```python
from build123d import *

# Parameters (mm, degrees)
BOSS_EXTRUDE1_DEPTH              = 5
SKETCH3_W                        = 11
SKETCH3_H                        = 5
BOSS_EXTRUDE2_DEPTH              = 5
SKETCH4_W                        = 5
SKETCH4_H                        = 5
BOSS_EXTRUDE3_DEPTH              = 21
SKETCH5_W                        = 10
SKETCH5_H                        = 5
BOSS_EXTRUDE4_DEPTH              = 20
SKETCH6_W                        = 11
SKETCH6_H                        = 5
BOSS_EXTRUDE5_DEPTH              = 5
SKETCH7_W                        = 5
SKETCH7_H                        = 5
BOSS_EXTRUDE6_DEPTH              = 21
SKETCH8_W                        = 10
SKETCH8_H                        = 5
BOSS_EXTRUDE7_DEPTH              = 20
SKETCH11_W                       = 10
SKETCH11_H                       = 5
BOSS_EXTRUDE8_DEPTH              = 3.5
SKETCH12_W                       = 10
SKETCH12_H                       = 5
BOSS_EXTRUDE9_DEPTH              = 3.5
CUT_EXTRUDE6_DEPTH               = 14.5
CUT_EXTRUDE8_DEPTH               = 41.078048855
CUT_EXTRUDE8_DEPTH_BACK          = 14.5
SKETCH17_W                       = 1.38
SKETCH17_H                       = 3.56
CUT_EXTRUDE9_DEPTH               = 14.5
CUT_EXTRUDE10_DEPTH              = 14.5
SKETCH_1_W                       = 8
SKETCH_1_H                       = 25
EXTRUDE_1_DEPTH                  = 5
SKETCH_2_W                       = 8
SKETCH_2_H                       = 25
EXTRUDE_2_DEPTH                  = 5
SKIZZE1_R                        = 1.5
SCHNITT_LINEAR_AUSTRAGEN1_DEPTH  = 10
AUFSATZ_LINEAR_AUSTRAGEN1_DEPTH  = 4
SKIZZE3_W                        = 10
SKIZZE3_H                        = 5
SCHNITT_LINEAR_AUSTRAGEN2_DEPTH  = 3.5
SCHNITT_LINEAR_AUSTRAGEN3_DEPTH  = 4
AUFSATZ_LINEAR_AUSTRAGEN3_DEPTH  = 11
SKIZZE7_R                        = 1.5
SCHNITT_LINEAR_AUSTRAGEN6_DEPTH  = 10
SKIZZE8_W                        = 10
SKIZZE8_H                        = 5
SCHNITT_LINEAR_AUSTRAGEN8_DEPTH  = 4
AUFSATZ_LINEAR_AUSTRAGEN4_DEPTH  = 4
SCHNITT_LINEAR_AUSTRAGEN9_DEPTH  = 4
AUFSATZ_LINEAR_AUSTRAGEN6_DEPTH  = 11
SKIZZE12_R                       = 1.5
SCHNITT_LINEAR_AUSTRAGEN10_DEPTH = 11


with BuildPart() as part:
    # Sketch1 → Boss-Extrude1 (new body)
    with BuildSketch(Plane(origin=(0, 0, 0), x_dir=(1, 0, 0), z_dir=(0, 1, 0))):
        Polygon((5.5, 3), (5.5, 0), (5.5, -3), (5.5, -8.5), (0, -8.5), (-5.5, -8.5), (-5.5, -3), (-5.5, 8.5), (0, 8.5), (5.5, 8.5), align=None)
    extrude(amount=BOSS_EXTRUDE1_DEPTH)

    # Sketch3 → Boss-Extrude2 (add)
    with BuildSketch(Plane.XY.offset(8.5)):
        with Locations((0, 2.5)):
            Rectangle(SKETCH3_W, SKETCH3_H)
    extrude(amount=BOSS_EXTRUDE2_DEPTH)

    # Sketch4 → Boss-Extrude3 (add)
    with BuildSketch(Plane(origin=(5.5, 0, 0), x_dir=(0, 0, -1), z_dir=(1, 0, 0))):
        with Locations((-11, 2.5)):
            Rectangle(SKETCH4_W, SKETCH4_H)
    extrude(amount=BOSS_EXTRUDE3_DEPTH)

    # Sketch5 → Boss-Extrude4 (add)
    with BuildSketch(Plane.XZ):
        with Locations((21.5, 11)):
            Rectangle(SKETCH5_W, SKETCH5_H)
    extrude(amount=BOSS_EXTRUDE4_DEPTH)

    # Sketch6 → Boss-Extrude5 (add)
    with BuildSketch(Plane(origin=(0, 0, -8.5), x_dir=(-1, 0, 0), z_dir=(0, 0, -1))):
        with Locations((0, 2.5)):
            Rectangle(SKETCH6_W, SKETCH6_H)
    extrude(amount=BOSS_EXTRUDE5_DEPTH)

    # Sketch7 → Boss-Extrude6 (add)
    with BuildSketch(Plane(origin=(5.5, 0, 0), x_dir=(0, 0, -1), z_dir=(1, 0, 0))):
        with Locations((11, 2.5)):
            Rectangle(SKETCH7_W, SKETCH7_H)
    extrude(amount=BOSS_EXTRUDE6_DEPTH)

    # Sketch8 → Boss-Extrude7 (add)
    with BuildSketch(Plane(origin=(0, 0, 0), x_dir=(-1, 0, 0), z_dir=(0, -1, 0))):
        with Locations((-21.5, 11)):
            Rectangle(SKETCH8_W, SKETCH8_H)
    extrude(amount=BOSS_EXTRUDE7_DEPTH)

    # Sketch11 → Boss-Extrude8 (add)
    with BuildSketch(Plane(origin=(0, 0, 8.5), x_dir=(-1, 0, 0), z_dir=(0, 0, -1))):
        with Locations((-21.5, -12.5)):
            Rectangle(SKETCH11_W, SKETCH11_H)
    extrude(amount=BOSS_EXTRUDE8_DEPTH)

    # Sketch12 → Boss-Extrude9 (add)
    with BuildSketch(Plane.XY.offset(-8.5)):
        with Locations((21.5, -12.5)):
            Rectangle(SKETCH12_W, SKETCH12_H)
    extrude(amount=BOSS_EXTRUDE9_DEPTH)

    # Sketch14 → Cut-Extrude6 (cut)
    with BuildSketch(Plane(origin=(26.5, 0, 0), x_dir=(0, 0, -1), z_dir=(1, 0, 0))):
        Polygon((-6.379568334, -12.879568334), (-6.379568334, -15), (-5, -15), (-5, -11.439784167), (-6.379568334, -11.439784167), align=None)
    extrude(amount=-CUT_EXTRUDE6_DEPTH, mode=Mode.SUBTRACT)

    # Sketch16 → Cut-Extrude8 (cut, two sides: drawn at the far end of the back side and taken through both)
    with BuildSketch(Plane(origin=(26.5, 0, 0), x_dir=(0, 0, -1), z_dir=(1, 0, 0)).offset(-CUT_EXTRUDE8_DEPTH_BACK)):
        Polygon((-6.379568334, -13), (-8.5, -15), (-7.439784167, -15), (-6.379568334, -15), align=None)
    extrude(amount=CUT_EXTRUDE8_DEPTH + CUT_EXTRUDE8_DEPTH_BACK, mode=Mode.SUBTRACT)

    # Sketch17 → Cut-Extrude9 (cut)
    with BuildSketch(Plane(origin=(26.5, 0, 0), x_dir=(0, 0, -1), z_dir=(1, 0, 0))):
        with Locations((5.69, -13.22)):
            Rectangle(SKETCH17_W, SKETCH17_H)
    extrude(amount=-CUT_EXTRUDE9_DEPTH, mode=Mode.SUBTRACT)

    # Sketch18 → Cut-Extrude10 (cut)
    with BuildSketch(Plane(origin=(26.5, 0, 0), x_dir=(0, 0, -1), z_dir=(1, 0, 0))):
        Polygon((6.38, -13), (6.38, -15), (8.5, -15), align=None)
    extrude(amount=-CUT_EXTRUDE10_DEPTH, mode=Mode.SUBTRACT)

    # 草图1 → 凸台-拉伸1 (add)
    with BuildSketch(Plane.XY.offset(13.5)):
        with Locations((30.5, -7.5)):
            Rectangle(SKETCH_1_W, SKETCH_1_H)
    extrude(amount=-EXTRUDE_1_DEPTH)

    # 草图2 → 凸台-拉伸2 (add)
    with BuildSketch(Plane(origin=(0, 0, -13.5), x_dir=(-1, 0, 0), z_dir=(0, 0, -1))):
        with Locations((-30.5, -7.5)):
            Rectangle(SKETCH_2_W, SKETCH_2_H)
    extrude(amount=-EXTRUDE_2_DEPTH)

    # Skizze1 → Schnitt-Linear austragen1 (cut)
    with BuildSketch(Plane(origin=(0, 5, 0), x_dir=(1, 0, 0), z_dir=(0, 1, 0))):
        with Locations(Location((-0.02687413, -4.000240759, 0), (0, 0, 270))):
            Circle(SKIZZE1_R)
        with Locations(Location((0.072523116, 4.001754227, 0), (0, 0, 270))):
            Circle(SKIZZE1_R)
    extrude(amount=-SCHNITT_LINEAR_AUSTRAGEN1_DEPTH, mode=Mode.SUBTRACT)

    # Skizze2 → Aufsatz-Linear austragen1 (add)
    with BuildSketch(Plane.XY.offset(13.5)):
        Polygon((-5.5, 5), (-5.5, 0), (16.5, 0), (16.5, -20), (34.5, -20), (34.5, 5), align=None)
    extrude(amount=AUFSATZ_LINEAR_AUSTRAGEN1_DEPTH)

    # Skizze3 → Schnitt-Linear austragen2 (cut)
    with BuildSketch(Plane(origin=(0, 0, 5), x_dir=(-1, 0, 0), z_dir=(0, 0, -1))):
        with Locations((-21.5, -12.5)):
            Rectangle(SKIZZE3_W, SKIZZE3_H)
    extrude(amount=-SCHNITT_LINEAR_AUSTRAGEN2_DEPTH, mode=Mode.SUBTRACT)

    # Skizze4 → Schnitt-Linear austragen3 (cut)
    with BuildSketch(Plane(origin=(0, 0, 8.5), x_dir=(-1, 0, 0), z_dir=(0, 0, -1))):
        Polygon((-34.5, 5), (-34.5, -20), (-16.5, -20), (-16.5, 0), (-5.5, 0), (-5.5, 5), align=None)
    extrude(amount=-SCHNITT_LINEAR_AUSTRAGEN3_DEPTH, mode=Mode.SUBTRACT)

    # Skizze6 → Aufsatz-Linear austragen3 (add)
    with BuildSketch(Plane.XY.offset(17.5)):
        Polygon((16, 5), (11, 5), (11, 0), (16.5, 0), (21, 0), (21, 5), align=None)
    extrude(amount=AUFSATZ_LINEAR_AUSTRAGEN3_DEPTH)

    # Skizze7 → Schnitt-Linear austragen6 (cut)
    with BuildSketch(Plane(origin=(0, 5, 0), x_dir=(1, 0, 0), z_dir=(0, 1, 0))):
        with Locations(Location((16, -23, 0), (0, 0, 270))):
            Circle(SKIZZE7_R)
    extrude(amount=-SCHNITT_LINEAR_AUSTRAGEN6_DEPTH, mode=Mode.SUBTRACT)

    # Skizze8 → Schnitt-Linear austragen8 (cut)
    with BuildSketch(Plane.XY.offset(-8.5)):
        with Locations((21.5, -12.5)):
            Rectangle(SKIZZE8_W, SKIZZE8_H)
    extrude(amount=SCHNITT_LINEAR_AUSTRAGEN8_DEPTH, mode=Mode.SUBTRACT)

    # Skizze9 → Aufsatz-Linear austragen4 (add)
    with BuildSketch(Plane(origin=(0, 0, -13.5), x_dir=(-1, 0, 0), z_dir=(0, 0, -1))):
        Polygon((-34.5, 5), (-34.5, -20), (-16.5, -20), (-16.5, 0), (5.5, 0), (5.5, 5), align=None)
    extrude(amount=AUFSATZ_LINEAR_AUSTRAGEN4_DEPTH)

    # Skizze10 → Schnitt-Linear austragen9 (cut)
    with BuildSketch(Plane.XY.offset(-8.5)):
        Polygon((5.5, 5), (5.5, 0), (16.5, 0), (16.5, -20), (34.5, -20), (34.5, 5), align=None)
    extrude(amount=-SCHNITT_LINEAR_AUSTRAGEN9_DEPTH, mode=Mode.SUBTRACT)

    # Skizze11 → Aufsatz-Linear austragen6 (add)
    with BuildSketch(Plane(origin=(0, 0, -17.5), x_dir=(-1, 0, 0), z_dir=(0, 0, -1))):
        Polygon((-11, 0), (-11, 5), (-21, 5), (-21, 0), (-16.5, 0), align=None)
    extrude(amount=AUFSATZ_LINEAR_AUSTRAGEN6_DEPTH)

    # Skizze12 → Schnitt-Linear austragen10 (cut)
    with BuildSketch(Plane(origin=(0, 5, 0), x_dir=(1, 0, 0), z_dir=(0, 1, 0))):
        with Locations(Location((16, 23, 0), (0, 0, 270))):
            Circle(SKIZZE12_R)
    extrude(amount=-SCHNITT_LINEAR_AUSTRAGEN10_DEPTH, mode=Mode.SUBTRACT)


solid = part.part
```
The model under review builds one solid part; all positions refer to its coordinate system, in mm. A direction names the side the tool comes from. Coordinates: 2 decimals unless noted, no trailing zeros. Loops run counter-clockwise (first coordinate to the right, second up) from the corner with the lowest first, then second, coordinate; pieces in that order, holes last. Notation, with made-up numbers: (69, 78.25) -> (80, 78.25) arc R26 ccw to (80, 110.25) -> close; hole circle Ø6 at (19, 84). An arc over 180 degrees is marked (long way). Answer as CSV lines item,"result".
Item 1: Take a section at A-A, the plane z = 23. State the section outline as (x, y) points, and give its area (3 significant figures).
Results below:
outline,"(11, 0) -> (14.5, 0) -> (14.5, 5) -> (11, 5) -> close; (17.5, 0) -> (21, 0) -> (21, 5) -> (17.5, 5) -> close"
area,"35.0 mm2"
Item 2: For L1, parallel to Z at x = 24, y = -17.5; L2, parallel to X at y = 3.25, z = 26; L3, parallel to Y at x = 12, z = 24.5, list the stretches that pass through material, from the lowest coordinate up.
Results below:
L1,"z = -17.5 to -12.5, 12.5 to 17.5"
L2,"x = 11 to 21"
L3,"y = 0 to 5"
Item 3: Take a section at C-C, the plane x = 4.5. State the section outline as (y, z) points, and give its area (3 significant figures).
Results below:
outline,"(0, -17.5) -> (5, -17.5) -> (5, 17.5) -> (0, 17.5) -> close"
area,"175 mm2"
Item 4: Draft analysis for pull direction Z (two halves, no side actions). For faces 6 (the flat face through (5.5, 2, 0)), 7 (the flat face through (3, 3, -17.5)), 8 (the flat face through (21, 2, 23)), state which applies: +Z half, -Z half, draft (parallel to the pull), parting line (faces both ways), or undercut.
Results below:
face 6,"undercut"
face 7,"-Z half"
face 8,"draft"
Item 5: Take a section at D-D, the plane z = 11. State the section outline as (x, y) points.
Results below:
outline,"(-5.5, 0) -> (5.5, 0) -> (5.5, 5) -> (-5.5, 5) -> close"
Item 6: Insertion check: pin 1 (5.5 mm diameter, centred on y = 2.5, z = -23.5, fed in from +X); pin 2 (5.5 mm diameter, centred on x = 29.5, y = -7.5, fed in from -Z); pin 3 (4 mm diameter, centred on x = 16, z = -23, fed in from -Y). Each pin has a flat end and moves straight along its axis. Give the tip position at first contact, or say it passes through.
Results below:
pin 1,"stops at x = 21"
pin 2,"stops at z = -17.5"
pin 3,"stops at y = 0"
Item 7: Take a section at B-B, the plane y = -12.5. State the section outline as (x, z) points, and give its area (3 significant figures).
Results below:
outline,"(16.5, -17.5) -> (34.5, -17.5) -> (34.5, -12.5) -> (16.5, -12.5) -> close; (16.5, 12.5) -> (34.5, 12.5) -> (34.5, 17.5) -> (16.5, 17.5) -> close"
area,"180 mm2"
Item 8: Machinability: for faces 1 (the flat face through (23, -7, 12.5)), 2 (the flat face through (11, 3, 23)), 3 (the flat face through (16.5, -10, -15)), 4 (the flat face through (11, 2, -23)), 5 (the flat face through (21, 3, -23)), which of the approach directions +Z, -Z, +X, -X, +Y, -Y give a long, thin tool a straight path to every point of the face, cutting with its end or side? Answer none if there is none.
Results below:
face 1,"+X, +Y, -Y"
face 2,"+Z, -X, +Y, -Y"
face 3,"+Z, -Z, -X, -Y"
face 4,"-Z, -X, +Y, -Y"
face 5,"-Z, +X, +Y, -Y"
